Autodesk Inventor part; units mm, degrees
ref_plane "YZ Plane" through (0, 0, 0) normal (1, 0, 0) x (0, 1, 0)
ref_plane "XZ Plane" through (0, 0, 0) normal (0, 1, 0) x (-1, 0, 0)
ref_plane "XY Plane" through (0, 0, 0) normal (0, 0, 1) x (1, 0, 0)
sketch "Sketch1" plane through (0, 0, 0) normal (0, 1, 0) x (-1, 0, 0)
  line L0 (0, 25.4) -> (25.4, 25.4)
  line L1 (25.4, 25.4) -> (25.4, 0)
  line L2 (25.4, 0) -> (0, 0)
  line L3 (0, 0) -> (0, 25.4)
  line L4 (22.225, 22.225) -> (3.175, 22.225)
  line L5 (3.175, 22.225) -> (3.175, 3.175)
  line L6 (3.175, 3.175) -> (22.225, 3.175)
  line L7 (22.225, 3.175) -> (22.225, 22.225)
  dimension "d0" = 25.4
  dimension "d1" = 25.4
  dimension "d2" = 3.175
extrude "Extrusion1" add sketch "Sketch1" along normal blind 177.8
sketch "Sketch2" plane through (-25.4, 0, 0) normal (-1, 0, 0) x (0, 0, 1)
  line L0 (0, 177.8) -> (25.4, 177.8)
  line L1 (25.4, 0) -> (0, 0)
  line L2 (12.7, 177.8) -> (12.7, 0) construction
  circle A0 centre (12.7, 165.1) radius 3.302
  circle A1 centre (12.7, 107.95) radius 3.302
  circle A2 centre (12.7, 152.4) radius 3.302
  circle A3 centre (12.7, 25.4) radius 3.302
  circle A4 centre (12.7, 9.525) radius 3.302
  dimension "d17" = 6.604
  dimension "d18" = 6.604
  dimension "d19" = 107.95
  dimension "d20" = 6.604
  dimension "d21" = 12.7
  dimension "d22" = 12.7
extrude "Extrusion2" cut sketch "Sketch2" against normal blind 25.4 contours A0 | A1 | A3 | A4
sketch "Sketch3" plane through (-25.4, 0, 0) normal (-1, 0, 0) x (0, 0, 1)
  circle A0 centre (12.7, 25.4) radius 3.302
  line L0 (25.4, 0) -> (0, 0)
  line L1 (0, 177.8) -> (25.4, 177.8)
  line L2 (12.7, 177.8) -> (12.7, 0) construction
  circle A1 centre (12.7, 50.8) radius 3.302
  circle A2 centre (12.7, 69.85) radius 3.302
  circle A3 centre (12.7, 88.9) radius 3.302
  circle A4 centre (12.7, 107.95) radius 3.302 construction
  circle A5 centre (12.7, 127) radius 3.302
  circle A6 centre (12.7, 146.05) radius 3.302
  dimension "d23" = 6.604
  dimension "d25" = 25.4
  dimension "d28" = 19.05
extrude "Extrusion3" cut sketch "Sketch3" against normal blind 25.4 contours A1 | A2 | A3 | A5 | A6
sketch "Sketch4" plane through (-25.4, 0, 25.4) normal (0, 0, 1) x (1, 0, 0)
  line L0 (25.4, 0) -> (0, 0)
  line L1 (0, 177.8) -> (25.4, 177.8)
  circle A0 centre (12.7, 139.7) radius 3.302
  line L2 (12.7, 177.8) -> (12.7, 0) construction
  circle A1 centre (12.7, 114.3) radius 3.302
  circle A2 centre (12.7, 88.9) radius 3.302
  circle A3 centre (12.7, 63.5) radius 3.302
  circle A4 centre (12.7, 38.1) radius 3.302
  dimension "d35" = 38.1
  dimension "d36" = 6.604
  dimension "d39" = 25.4
extrude "Extrusion4" cut sketch "Sketch4" against normal blind 25.4 contours A0 | A3 | A4
equation "\"d20\" = d17"
equation "\"d22\" = d21"
properties part number "Chassis V1.500 Part3-mirror" material "Aluminum 6061"
Verification items for the finished model (mm, model axes). Coordinates: 2 decimals unless noted, no trailing zeros. Order: outer loops, then holes, each group sorted by start corner. A loop starts at its lowest first (then second) coordinate and runs counter-clockwise, first axis right, second up.
Item 1: Section check B-B, the plane x = -18. Enter the section's corners in (y, z) (3 decimals), then the cut area to 3 significant figures.
Filled in:
outline: (0, 0) - (177.8, 0) - (177.8, 3.175) - (0, 3.175) - close; (0, 22.225) - (177.8, 22.225) - (177.8, 25.4) - (0, 25.4) - close
area: 1,130 mm2
Item 2: Release check for a two-part mould opening along X. For faces 1 (the face through (-25.4, 88, 19)), 2 (the face through (-13, 88, 3.175)), 3 (the face through (-23.835, 66.627, 11.984)) record: +X half, -X half, draft (parallel to the pull), parting line (faces both ways), or undercut.
Filled in:
face 1: -X half
face 2: undercut
face 3: draft
Item 3: Section check D-D, the plane y = 97.5. Enter the section's corners in (x, z) (3 decimals), then the cut area to 3 significant figures.
Filled in:
outline: (-25.4, 0) - (0, 0) - (0, 25.4) - (-25.4, 25.4) - close; hole (-22.225, 3.175) - (-3.175, 3.175) - (-3.175, 22.225) - (-22.225, 22.225) - close
area: 282 mm2
Item 4: Section check C-C, the plane y = 71.5. Enter the section's corners in (x, z) (3 decimals), then the cut area to 3 significant figures.
Filled in:
outline: (-25.4, 0) - (0, 0) - (0, 9.84) - (-3.175, 9.84) - (-3.175, 3.175) - (-22.225, 3.175) - (-22.225, 9.84) - (-25.4, 9.84) - close; (-25.4, 15.56) - (-22.225, 15.56) - (-22.225, 22.225) - (-3.175, 22.225) - (-3.175, 15.56) - (0, 15.56) - (0, 25.4) - (-25.4, 25.4) - close
area: 246 mm2
Item 5: Material ranges on L1, parallel to X at y = 41, z = 18.5 (3 decimals); L2, parallel to Z at x = -3.75, y = 50.5 (3 decimals); L3, parallel to Y at x = -11, z = 23.5, recorded low to high.
Filled in:
L1: x = -25.4 to -22.225, -3.175 to 0
L2: z = 0 to 3.175, 22.225 to 25.4
L3: y = 0 to 35.27, 40.93 to 60.67, 66.33 to 136.87, 142.53 to 177.8
Item 6: Depth check by flat-ended pin: pin 1 (7.5 mm diameter, centred on x = -12.7, y = 38.1, fed in from +Z). Enter the tip coordinate at first touch or a pass-through.
Filled in:
pin 1: stops at z = 25.4
Item 7: Section check A-A, the plane z = 6.75. Enter the section's corners in (x, y) (3 decimals).
Filled in:
outline: (-25.4, 0) - (-22.225, 0) - (-22.225, 177.8) - (-25.4, 177.8) - close; (-3.175, 0) - (0, 0) - (0, 177.8) - (-3.175, 177.8) - close
